from build123d import *

# Parameters (mm, degrees)
SKETCH1_R                                     = 50.5
BOSS_EXTRUDE1_DEPTH                           = 60
SKETCH2_W                                     = 60
SKETCH2_H                                     = 115
BOSS_EXTRUDE2_DEPTH                           = 20
CIRPATTERN1_COUNT                             = 4
BOSS_EXTRUDE3_DEPTH                           = 20
FILLET1_R                                     = 9
BOSS_EXTRUDE4_DEPTH                           = 10
CIRPATTERN4_COUNT                             = 2
SKETCH9_W                                     = 20
SKETCH9_H                                     = 80
BOSS_EXTRUDE5_DEPTH                           = 40
FILLET2_R                                     = 20
CUT_EXTRUDE1_DEPTH                            = 8
CUT_EXTRUDE2_DEPTH                            = 203.255407839
CUT_EXTRUDE3_DEPTH                            = 15
CIRPATTERN5_COUNT                             = 4
SKETCH21_R                                    = 7.5
CUT_EXTRUDE4_DEPTH                            = 208.140652698
CUT_EXTRUDE4_DEPTH_BACK                       = 208.140652698
SKETCH22_R                                    = 10
CUT_EXTRUDE5_DEPTH                            = 204.303344783
CUT_EXTRUDE5_DEPTH_BACK                       = 204.303344783
CBORE_FOR_M12_HEX_HEAD_CAP_SCREW1_D           = 8
CBORE_FOR_M12_HEX_HEAD_CAP_SCREW1_CBORE_D     = 15
CBORE_FOR_M12_HEX_HEAD_CAP_SCREW1_CBORE_DEPTH = 7
RIB1_REACH                                    = 224.96
SKETCH17_WALL_W                               = 513.393885606
SKETCH17_WALL_H                               = 10


with BuildPart() as part:
    # Sketch1 → Boss-Extrude1 (new body)
    with BuildSketch(Plane(origin=(0, 0, 0), x_dir=(1, 0, 0), z_dir=(0, 1, 0))):
        with Locations(Location((0, 0, 0), (0, 0, 270))):
            Circle(SKETCH1_R)
    extrude(amount=BOSS_EXTRUDE1_DEPTH)

    # Sketch2 → Boss-Extrude2 (add)
    with BuildSketch(Plane.XZ):
        with Locations((0, 57.5)):
            Rectangle(SKETCH2_W, SKETCH2_H)
    boss_extrude2 = extrude(amount=-BOSS_EXTRUDE2_DEPTH)

    # CirPattern1: Boss-Extrude2 ×4 about axis, 1 skipped
    cirpattern1_axis = Axis((0, 0, 0), (0, -1, 0))
    add([boss_extrude2.rotate(cirpattern1_axis, i * 360 / CIRPATTERN1_COUNT) for i in range(1, CIRPATTERN1_COUNT) if i not in (2,)])

    # Sketch4 → Boss-Extrude3 (add)
    with BuildSketch(Plane(origin=(0, 60, 0), x_dir=(1, 0, 0), z_dir=(0, 1, 0))):
        with BuildLine():
            Line((-49.957724584, 7.380769231), (-31.161748998, 134.603846154))
            ThreePointArc((-31.161748998, 134.603846154), (0, 161.5), (31.161748998, 134.603846154))
            Line((31.161748998, 134.603846154), (49.957724584, 7.380769231))
            ThreePointArc((49.957724584, 7.380769231), (0, -50.5), (-49.957724584, 7.380769231))
        make_face()
    extrude(amount=-BOSS_EXTRUDE3_DEPTH)

    # Fillet1
    fillet1_edges = [part.edges().sort_by_distance(p)[0] for p in [
        (30, 10, 115),
        (-30, 10, 115),
        (-115, 10, 30),
        (-115, 10, -30),
        (115, 10, -30),
        (115, 10, 30),
    ]]
    fillet(fillet1_edges, radius=FILLET1_R)

    # Sketch8 → Boss-Extrude4 (add, symmetric)
    with BuildSketch(Plane.XY):
        with BuildLine():
            Line((-115, 20), (-115, 40))
            ThreePointArc((-115, 40), (-109.142135624, 54.142135624), (-95, 60))
            Line((-95, 60), (-45, 60))
            Line((-45, 60), (-45, 20))
            Line((-45, 20), (-115, 20))
        make_face()
    boss_extrude4 = extrude(amount=BOSS_EXTRUDE4_DEPTH, both=True)

    # CirPattern4: Boss-Extrude4 ×2 about axis
    cirpattern4_axis = Axis((0, -13.978729863, 0), (0, 1, 0))
    for i in range(1, CIRPATTERN4_COUNT):
        add(boss_extrude4.rotate(cirpattern4_axis, i * 360 / CIRPATTERN4_COUNT))

    # Sketch9 → Boss-Extrude5 (add)
    with BuildSketch(Plane(origin=(0, 20, 0), x_dir=(1, 0, 0), z_dir=(0, 1, 0))):
        with Locations((0, -75)):
            Rectangle(SKETCH9_W, SKETCH9_H)
    extrude(amount=BOSS_EXTRUDE5_DEPTH)

    # Fillet2
    fillet2_edges = [part.edges().sort_by_distance(p)[0] for p in [
        (0, 60, 115),
    ]]
    fillet(fillet2_edges, radius=FILLET2_R)

    # Sketch19 → Cut-Extrude1 (cut)
    with BuildSketch(Plane(origin=(0, 60, 0), x_dir=(1, 0, 0), z_dir=(0, 1, 0))):
        with BuildLine():
            ThreePointArc((-43, 0), (-32, -11), (-21, 0))
            ThreePointArc((-21, 0), (0, 21), (21, 0))
            ThreePointArc((21, 0), (32, -11), (43, 0))
            ThreePointArc((43, 0), (0, 43), (-43, 0))
        make_face()
    extrude(amount=-CUT_EXTRUDE1_DEPTH, mode=Mode.SUBTRACT)

    # Sketch6 → Cut-Extrude2 (cut, symmetric)
    with BuildSketch(Plane(origin=(0, 20, 0), x_dir=(1, 0, 0), z_dir=(0, 1, 0))):
        with BuildLine():
            Line((25, -75), (25, -91))
            ThreePointArc((25, -91), (20, -96), (15, -91))
            Line((15, -91), (15, -75))
            ThreePointArc((15, -75), (20, -70), (25, -75))
        make_face()
        with BuildLine():
            Line((-25, -75), (-25, -91))
            ThreePointArc((-25, -91), (-20, -96), (-15, -91))
            Line((-15, -91), (-15, -75))
            ThreePointArc((-15, -75), (-20, -70), (-25, -75))
        make_face()
    cut_extrude2 = extrude(amount=CUT_EXTRUDE2_DEPTH, both=True, mode=Mode.SUBTRACT)

    # Sketch20 → Cut-Extrude3 (cut)
    with BuildSketch(Plane(origin=(0, 60, 0), x_dir=(1, 0, 0), z_dir=(0, 1, 0))):
        with BuildLine():
            ThreePointArc((-19, 0), (0, 19), (19, 0))
            ThreePointArc((19, 0), (21.917140163, -8.205847762), (29.359375, -12.72898659))
            ThreePointArc((29.359375, -12.72898659), (0, -32), (-29.359375, -12.72898659))
            ThreePointArc((-29.359375, -12.72898659), (-21.917140163, -8.205847762), (-19, 0))
        make_face()
    extrude(amount=-CUT_EXTRUDE3_DEPTH, mode=Mode.SUBTRACT)

    # CirPattern5: Cut-Extrude2 ×4 about axis, 1 skipped
    cirpattern5_axis = Axis((0, 0, 0), (0, -1, 0))
    add([cut_extrude2.rotate(cirpattern5_axis, i * 360 / CIRPATTERN5_COUNT) for i in range(1, CIRPATTERN5_COUNT) if i not in (2,)], mode=Mode.SUBTRACT)

    # Sketch21 → Cut-Extrude4 (cut, two sides)
    with BuildSketch(Plane(origin=(0, 60, 0), x_dir=(1, 0, 0), z_dir=(0, 1, 0))) as cut_extrude4_sk:
        with Locations(Location((0, -32, 0), (0, 0, 270))):
            Circle(SKETCH21_R)
    extrude(amount=CUT_EXTRUDE4_DEPTH, mode=Mode.SUBTRACT)
    extrude(cut_extrude4_sk.sketch, amount=-CUT_EXTRUDE4_DEPTH_BACK, mode=Mode.SUBTRACT)

    # Sketch22 → Cut-Extrude5 (cut, two sides)
    with BuildSketch(Plane(origin=(0, 45, 0), x_dir=(1, 0, 0), z_dir=(0, 1, 0))) as cut_extrude5_sk:
        with Locations(Location((0, 0, 0), (0, 0, 270))):
            Circle(SKETCH22_R)
    extrude(amount=CUT_EXTRUDE5_DEPTH, mode=Mode.SUBTRACT)
    extrude(cut_extrude5_sk.sketch, amount=-CUT_EXTRUDE5_DEPTH_BACK, mode=Mode.SUBTRACT)

    # CBORE for M12 Hex Head Cap Screw1 (through all)
    with Locations(Plane(origin=(0, 52, 0), x_dir=(1, 0, 0), z_dir=(0, 1, 0))):
        with Locations((-32, 0), (32, 0), (0, 32)):
            CounterBoreHole(CBORE_FOR_M12_HEX_HEAD_CAP_SCREW1_D / 2, CBORE_FOR_M12_HEX_HEAD_CAP_SCREW1_CBORE_D / 2, CBORE_FOR_M12_HEX_HEAD_CAP_SCREW1_CBORE_DEPTH)

    # Sketch26 → Revolve1 (revolve)
    with BuildSketch(Plane(origin=(0, 0, 0), x_dir=(0, 0, -1), z_dir=(1, 0, 0))):
        Polygon((161.5, 60), (151.5, 102), (130, 102), (130, 60), align=None)
    revolve(axis=Axis((0, -4.416477213, -130), (0, 1, 0)))

    # Sketch17 wall → Rib1 (add, up to next)
    with BuildSketch(Plane(origin=(0, 77.5, -79.166666666), x_dir=(0, -0.534567509226, 0.845125776485), z_dir=(0, -0.845125776485, -0.534567509226)), mode=Mode.PRIVATE) as rib1_sk1:
        Rectangle(SKETCH17_WALL_W, SKETCH17_WALL_H)
    rib1_tool1 = extrude(rib1_sk1.sketch, amount=RIB1_REACH, mode=Mode.PRIVATE) - part.part
    add(rib1_tool1.solids().sort_by_distance((0, 77.5, -79.166666666))[0])

    # Sketch27 → Cut-Revolve1 (revolve, cut)
    with BuildSketch(Plane(origin=(0, 0, 0), x_dir=(0, 0, -1), z_dir=(1, 0, 0)), mode=Mode.PRIVATE) as cut_revolve1_sk:
        Polygon((142.5, 102), (152.5, 40), (130, 40), (130, 102), align=None)
    revolve(cut_revolve1_sk.sketch.rotate(Axis((0, 116.719168037, -130), (0, -1, 0)), 180), axis=Axis((0, 116.719168037, -130), (0, -1, 0)), mode=Mode.SUBTRACT)


solid = part.part
Source: CAD feature listing. Evaluate the final solid. Frame: model axes, mm. A direction names the side the tool comes from. Give positions to 0.01 mm unless a question says otherwise; leave off trailing zeros. Write each loop counter-clockwise with the first axis right and the second up, starting at its lowest first coordinate (ties: lowest second). Pieces come first, ordered by that corner, then holes. Notation, with made-up numbers: (64.5, 28) -> (93.5, 28) arc R15 ccw to (93.5, 42) -> close; hole circle Ø3 at (47, 59.5). An arc over 180 degrees is marked (long way). Write item = value, one per line.
Q1. Line query: line 1 (X direction, y = 5.5, z = -3.5); line 2 (X direction, y = 32, z = 95.5). Output: solid intervals per line, ascending. Write a range as from..to.
Here are the results:
line_1 = -115..-33.94, -30.06..-9.37, 9.37..30.06, 33.94..115
line_2 = -10..10
Q2. Cut plane B-B on y = 36.5. Return loops of the section in (x, z).
Here are the results:
outline = (-115, -10) -> (-49.5, -10) arc R50.5 ccw to (49.5, -10) -> (115, -10) -> (115, 10) -> (49.5, 10) arc R50.5 ccw to (10, 49.5) -> (10, 115) -> (-10, 115) -> (-10, 49.5) arc R50.5 ccw to (-49.5, 10) -> (-115, 10) -> close; hole circle Ø8 at (-32, 0); hole circle Ø20 at (0, 0); hole circle Ø15 at (0, 32); hole circle Ø8 at (0, -32); hole circle Ø8 at (32, 0)
Q3. Mould query, pull axis Z, two halves, no side actions, for faces 5 (the face through (82, 40, -10)), 6 (the face through (0, 60, -46)), 7 (the face through (20, 10, 70)), 8 (the face through (-27.294, 10.14, 112.434)). Classes: +Z half, -Z half, draft (parallel to the pull), parting line (faces both ways), or undercut.
Here are the results:
face_5 = -Z half
face_6 = draft
face_7 = undercut
face_8 = +Z half
Q4. Reachability of faces 1 (the face through (78, 20, 27)), 2 (the face through (112.294, 10.14, 27.434)), 3 (the face through (-39.493, 48.549, -0.33)), 4 (the face through (-96, 10, 20)) from +Z, -Z, +X, -X, +Y, -Y: full face, straight path, thin tool, end or side. Return the list, or none.
Here are the results:
face_1 = +Z, +X, +Y
face_2 = +Z, +X, +Y, -Y
face_3 = +Y
face_4 = +Y, -Y
Q5. First-contact query: pin 1 (13 mm diameter, centred on y = 11.5, z = 85, fed in from +X); pin 2 (22 mm diameter, centred on x = 92, z = 22, fed in from +Y); pin 3 (17 mm diameter, centred on x = 32, z = 0, fed in from -Y); pin 4 (6 mm diameter, centred on x = -5.5, y = 33, fed in from -Z). Flat tips, straight axial feed; report the tip coordinate or a pass-through.
Here are the results:
pin_1 = 30
pin_2 = 20
pin_3 = 0
pin_4 = -50.44
Q6. Cut plane D-D on y = 87.5. Return loops of the section in (x, z).
Here are the results:
outline = (-5, -105.55) arc R24.95 ccw (long way) to (5, -105.55) -> (5, -94.98) -> (-5, -94.98) -> close; hole circle Ø29.68 at (0, -130)
Q7. Cut plane C-C on y = 10. State how many separate pieces and enclosed holes the cut face has, then the cut area to 3 significant figures.
Here are the results:
separate_pieces = 1
enclosed_holes = 11
area = 18,000 mm²
Q8. Cut plane A-A on z = 83.5. Return loops of the section in (x, y).
Here are the results:
outline = (-30, 0) -> (-25, 0) -> (-25, 20) -> (-30, 20) -> close; (-15, 0) -> (15, 0) -> (15, 20) -> (10, 20) -> (10, 60) -> (-10, 60) -> (-10, 20) -> (-15, 20) -> close; (25, 0) -> (30, 0) -> (30, 20) -> (25, 20) -> close
